```python
from build123d import *

# Parameters (mm, degrees)
SKETCH_1_R          = 24
SKETCH_1_R_2        = 3.25
EXTRUDE_1_DEPTH     = 15.5
SKETCH_2_R          = 19.5
SKETCH_2_R_2        = 10
CUT_EXTRUDE_1_DEPTH = 10.5
CUT_EXTRUDE_2_DEPTH = 20


with BuildPart() as part:
    # Эскиз1 → Вытянуть1 (new body)
    with BuildSketch(Plane.XY):
        Circle(SKETCH_1_R)
        with Locations(Location((0, 0, 0), (0, 0, 180))):
            Circle(SKETCH_1_R_2, mode=Mode.SUBTRACT)
    extrude(amount=EXTRUDE_1_DEPTH)

    # Эскиз2 → Вырез-Вытянуть1 (cut)
    with BuildSketch(Plane.XY.offset(15.5)):
        Circle(SKETCH_2_R)
        Circle(SKETCH_2_R_2, mode=Mode.SUBTRACT)
    extrude(amount=-CUT_EXTRUDE_1_DEPTH, mode=Mode.SUBTRACT)

    # Эскиз3 → Вырез-Вытянуть2 (cut)
    with BuildSketch(Plane(origin=(0, 0, 0), x_dir=(-1, 0, 0), z_dir=(0, 0, -1))):
        with BuildLine():
            Line((3, 20), (3, 23.8117618))
            ThreePointArc((3, 23.8117618), (0, 24), (-3, 23.8117618))
            Line((-3, 23.8117618), (-3, 20))
            ThreePointArc((-3, 20), (0, 17), (3, 20))
        make_face()
        with BuildLine():
            Line((3, -20), (3, -23.8117618))
            ThreePointArc((3, -23.8117618), (0, -24), (-3, -23.8117618))
            Line((-3, -23.8117618), (-3, -20))
            ThreePointArc((-3, -20), (0, -17), (3, -20))
        make_face()
    extrude(amount=-CUT_EXTRUDE_2_DEPTH, mode=Mode.SUBTRACT)


solid = part.part
```
Verification items for the finished model (mm, model axes). A direction names the side the tool comes from. Round coordinates to 2 decimals unless told otherwise and drop trailing zeros. Write each loop counter-clockwise with the first axis right and the second up, starting at its lowest first coordinate (ties: lowest second). Pieces come first, ordered by that corner, then holes.
1. Access from +Z, -Z, +X, -X, +Y, -Y to the whole of each face (thin tool, end or side, straight path). Record for faces 5 (the flat face through (20, 2, 15.5)), 6 (the flat face through (-3, -22, 8)), 7 (the flat face through (3, 22, 8)), 8 (the cylindrical face through (-2.17, -9.76, 10.32)).
2. Scan lines: L1, parallel to Y at x = 0, z = 9.5; L2, parallel to Y at x = 9, z = 12; L3, parallel to Y at x = -6, z = 9.25. Record each from-to range of solid material in increasing order.
3. Section check D-D on z = 2.5. Enter the section's corners in (x, y), plus the area to 3 significant figures.
4. Section check C-C on y = 0. Enter the section's corners in (x, z), plus the area to 3 significant figures.
5. Section check A-A on z = 13.25. Enter the section's corners in (x, y), plus the area to 3 significant figures.
6. Section check B-B on x = 0. Enter the section's corners in (y, z), plus the area to 3 significant figures.
7. Gauge pin test, flat ends, axial feed: P1, Ø3, axis at x = 15, z = 8, coming from the +Y side; P2, Ø3, axis at y = -22, z = 6.5, coming from the -X side; P3, Ø6, axis at y = 18, z = 13, coming from the -X side (3 decimals). Record the tip position at first contact, or that the pin passes through.
8. Draft check along Y on faces 1 (the flat face through (-20, 2, 15.5)), 2 (the cylindrical face through (0, -17, 4)), 3 (the cylindrical face through (24, 0, 8)), 4 (the flat face through (-9, 5, 5)). Enter one of: +Y half, -Y half, draft (parallel to the pull), parting line (faces both ways), or undercut.
Answer:
1. face 5: +Z, +X, -X, +Y, -Y
1. face 6: +Z, -Z, -Y
1. face 7: +Z, -Z, +Y
1. face 8: +Z
2. L1: y = -10 to -3.25, 3.25 to 10
2. L2: y = -22.25 to -17.3, -4.36 to 4.36, 17.3 to 22.25
2. L3: y = -23.24 to -18.55, -8 to 8, 18.55 to 23.24
3. outline: (-3, -23.81) - (-3, -20) arc R3 cw to (3, -20) - (3, -23.81) arc R24 ccw to (3, 23.81) - (3, 20) arc R3 cw to (-3, 20) - (-3, 23.81) arc R24 ccw to start; hole circle Ø6.5 at (0, 0)
3. area: 1,700 mm2
4. outline: (-24, 0) - (-3.25, 0) - (-3.25, 15.5) - (-10, 15.5) - (-10, 5) - (-19.5, 5) - (-19.5, 15.5) - (-24, 15.5) - close; (3.25, 0) - (24, 0) - (24, 15.5) - (19.5, 15.5) - (19.5, 5) - (10, 5) - (10, 15.5) - (3.25, 15.5) - close
4. area: 444 mm2
5. outline: circle Ø20 at (0, 0); (-3, -23.81) - (-3, -20) arc R3 cw to (-2.91, -19.28) arc R19.5 cw to (-2.91, 19.28) arc R3 cw to (-3, 20) - (-3, 23.81) arc R24 ccw to start; (2.91, -19.28) arc R3 cw to (3, -20) - (3, -23.81) arc R24 ccw to (3, 23.81) - (3, 20) arc R3 cw to (2.91, 19.28) arc R19.5 cw to start; hole circle Ø6.5 at (0, 0)
5. area: 842 mm2
6. outline: (-17, 0) - (-3.25, 0) - (-3.25, 15.5) - (-10, 15.5) - (-10, 5) - (-17, 5) - close; (3.25, 0) - (17, 0) - (17, 5) - (10, 5) - (10, 15.5) - (3.25, 15.5) - close
6. area: 279 mm2
7. P1: stops at y = 19.84
7. P2: stops at x = -12.48
7. P3: stops at x = -18.735
8. face 1: draft
8. face 2: -Y half
8. face 3: parting line
8. face 4: undercut
